```python
from build123d import *

# Parameters (mm, degrees)
SKETCH1_W           = 60
SKETCH1_H           = 60
BOSS_EXTRUDE1_DEPTH = 60
CUT_EXTRUDE1_DEPTH  = 108
SKETCH2_R           = 4
CUT_EXTRUDE2_DEPTH  = 108
CUT_EXTRUDE3_DEPTH  = 30
SKETCH4_R           = 7.5
CUT_EXTRUDE4_DEPTH  = 5.5


with BuildPart() as part:
    # Sketch1 → Boss-Extrude1 (new body)
    with BuildSketch(Plane(origin=(0, 0, 0), x_dir=(1, 0, 0), z_dir=(0, 1, 0))):
        Rectangle(SKETCH1_W, SKETCH1_H)
    extrude(amount=BOSS_EXTRUDE1_DEPTH)

    # 3DSketch1 → Cut-Extrude1 (cut)
    with BuildSketch(Plane(origin=(-22, 60, -22), x_dir=(0.7071067811865481, 0, 0.707106781186547), z_dir=(0, 1, 0))):
        Polygon((0, 0), (31.112698372, -31.112698372), (62.225396744, 0), (31.112698372, 31.112698372), align=None)
    extrude(amount=-CUT_EXTRUDE1_DEPTH, mode=Mode.SUBTRACT)

    # Sketch2 → Cut-Extrude2 (cut)
    with BuildSketch(Plane.ZY.offset(-22)):
        with Locations((0, 30)):
            Circle(SKETCH2_R)
    extrude(amount=-CUT_EXTRUDE2_DEPTH, mode=Mode.SUBTRACT)

    # Sketch3 → Cut-Extrude3 (cut)
    with BuildSketch(Plane.ZY.offset(30)):
        with BuildLine():
            Line((-10.5, 40.5), (-10.5, 43.5))
            Line((-10.5, 43.5), (-7.5, 43.5))
            ThreePointArc((-7.5, 43.5), (-12.621320344, 45.621320344), (-10.5, 40.5))
        make_face()
        with BuildLine():
            Line((-7.5, 43.5), (-10.5, 43.5))
            Line((-10.5, 43.5), (-10.5, 40.5))
            ThreePointArc((-10.5, 40.5), (-8.378679656, 41.378679656), (-7.5, 43.5))
        make_face()
        with BuildLine():
            ThreePointArc((13.5, 43.5), (10.5, 46.5), (7.5, 43.5))
            Line((7.5, 43.5), (10.5, 43.5))
            Line((10.5, 43.5), (10.5, 40.5))
            ThreePointArc((10.5, 40.5), (12.621320344, 41.378679656), (13.5, 43.5))
        make_face()
        with BuildLine():
            Line((10.5, 43.5), (7.5, 43.5))
            ThreePointArc((7.5, 43.5), (8.378679656, 41.378679656), (10.5, 40.5))
            Line((10.5, 40.5), (10.5, 43.5))
        make_face()
        with BuildLine():
            ThreePointArc((13.5, 16.5), (12.621320344, 18.621320344), (10.5, 19.5))
            Line((10.5, 19.5), (10.5, 16.5))
            Line((10.5, 16.5), (7.5, 16.5))
            ThreePointArc((7.5, 16.5), (10.5, 13.5), (13.5, 16.5))
        make_face()
        with BuildLine():
            Line((10.5, 16.5), (10.5, 19.5))
            ThreePointArc((10.5, 19.5), (8.378679656, 18.621320344), (7.5, 16.5))
            Line((7.5, 16.5), (10.5, 16.5))
        make_face()
        with BuildLine():
            ThreePointArc((-7.5, 16.5), (-8.378679656, 18.621320344), (-10.5, 19.5))
            Line((-10.5, 19.5), (-10.5, 16.5))
            Line((-10.5, 16.5), (-7.5, 16.5))
        make_face()
        with BuildLine():
            Line((-10.5, 16.5), (-10.5, 19.5))
            ThreePointArc((-10.5, 19.5), (-12.621320344, 14.378679656), (-7.5, 16.5))
            Line((-7.5, 16.5), (-10.5, 16.5))
        make_face()
    extrude(amount=-CUT_EXTRUDE3_DEPTH, mode=Mode.SUBTRACT)

    # Sketch4 → Cut-Extrude4 (cut)
    with BuildSketch(Plane.ZY.offset(-22)):
        with Locations((0, 30)):
            Circle(SKETCH4_R)
    extrude(amount=-CUT_EXTRUDE4_DEPTH, mode=Mode.SUBTRACT)


solid = part.part
```
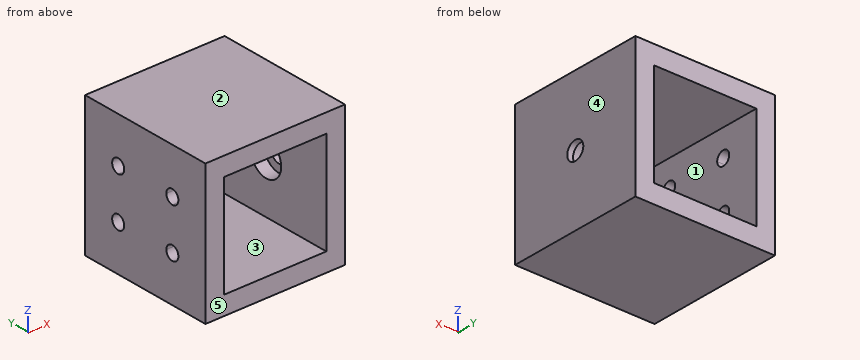
Check sheet for the modelled part. Datum: model origin and axes. Units: mm. Face numbers are marked on the shaded views. A direction names the side the tool comes from. Coordinates: 2 decimals unless noted, no trailing zeros. Write each loop counter-clockwise with the first axis right and the second up, starting at its lowest first coordinate (ties: lowest second). Pieces come first, ordered by that corner, then holes. Notation, with made-up numbers: (11.5, 63) -> (53.5, 63) arc R33 ccw to (53.5, 97) -> close; hole circle Ø7 at (27.25, 24.25). An arc over 180 degrees is marked (long way). Use a Markdown table: item, result.
1. Sectioned sample at C-C (z = 0). Enter the section's corners in (x, y), plus the area to 4 significant figures.
Reported:
| item | result |
|---|---|
| outline | (-30, 0) -> (-22, 0) -> (-22, 60) -> (-30, 60) -> close; (22, 0) -> (30, 0) -> (30, 26) -> (27.5, 26) -> (27.5, 22.5) -> (22, 22.5) -> close; (22, 37.5) -> (27.5, 37.5) -> (27.5, 34) -> (30, 34) -> (30, 60) -> (22, 60) -> close |
| area | 857.5 mm2 |
2. Sectioned sample at D-D (x = -23.5). Enter the section's corners in (y, z).
Reported:
| item | result |
|---|---|
| outline | (0, -30) -> (60, -30) -> (60, 30) -> (0, 30) -> close; hole circle Ø6 at (16.5, -10.5); hole circle Ø6 at (16.5, 10.5); hole circle Ø6 at (43.5, -10.5); hole circle Ø6 at (43.5, 10.5) |
3. Sectioned sample at B-B (y = 51). Enter the section's corners in (x, z), plus the area to 3 significant figures.
Reported:
| item | result |
|---|---|
| outline | (-30, -30) -> (30, -30) -> (30, 30) -> (-30, 30) -> close; hole (-22, -22) -> (22, -22) -> (22, 22) -> (-22, 22) -> close |
| area | 1,660 mm2 |
4. Go/stop test with a flat-tipped pin: pin 1 Ø8 at (y, z) = (16.5, -10.5) entering from -X. Record where the tip stops, or that it passes through.
Reported:
| item | result |
|---|---|
| pin 1 | stops at x = -30 |
5. Sectioned sample at A-A (x = -9.5). Enter the section's corners in (y, z), plus the area to 3 significant figures.
Reported:
| item | result |
|---|---|
| outline | (0, -30) -> (60, -30) -> (60, -22) -> (0, -22) -> close; (0, 22) -> (60, 22) -> (60, 30) -> (0, 30) -> close |
| area | 960 mm2 |
6. Tool access check on the marked faces 1 and 2. Record the directions out of +Z, -Z, +X, -X, +Y, -Y that give a thin tool (end or side, any length) a straight path to the whole face; none if there is none.
Reported:
| item | result |
|---|---|
| face 1 | +Y, -Y |
| face 2 | +Z, +X, -X, +Y, -Y |
7. Release check for a two-part mould opening along X. For the marked faces 3, 4 and 5 record: pulls with the +X half, pulls with the -X half, needs draft (parallel to the pull), parting line crosses it, or undercut.
Reported:
| item | result |
|---|---|
| face 3 | undercut |
| face 4 | pulls with the +X half |
| face 5 | needs draft |
8. Scan lines: line 1 along Z through (x, y) = (-24, 43.5); line 2 along Z through (x, y) = (17.5, 12.5). Record each from-to range of solid material in increasing order.
Reported:
| item | result |
|---|---|
| line 1 | z = -30 to -13.5, -7.5 to 7.5, 13.5 to 30 |
| line 2 | z = -30 to -22, 22 to 30 |
